Design review of the part built by this model. Coordinates are the model's own, in mm. A direction names the side the tool comes from. Give positions to 0.01 mm unless a question says otherwise; leave off trailing zeros. Loops run counter-clockwise (first coordinate to the right, second up) from the corner with the lowest first, then second, coordinate; pieces in that order, holes last.
from build123d import *

# Parameters (mm, degrees)
F0_W     = 51.3991490006
F0_H     = 50.7968105376
F0_R     = 5.0314784616
F1_DEPTH = 43.942
F2_W     = 28.5104624927
F2_H     = 18.070012331
F3_DEPTH = 25.908
F4_W     = 80.7127282023
F4_H     = 44.773478061
F5_DEPTH = 84.836


with BuildPart() as f1:
    # F0 (on Right) → F1 (new body, symmetric)
    with BuildSketch(Plane.YZ):
        with Locations((0, 25.3984052688)):
            Rectangle(F0_W, F0_H)
        with Locations((0, 25.3984052688)):
            Circle(F0_R, mode=Mode.SUBTRACT)
    extrude(amount=F1_DEPTH, both=True)

    # F2 (on Front) → F3 (cut, symmetric)
    with BuildSketch(Plane.XZ):
        with Locations((0, 41.862193495)):
            Rectangle(F2_W, F2_H)
    extrude(amount=F3_DEPTH, both=True, mode=Mode.SUBTRACT)

    # F4 (on Top) → F5 (cut)
    with BuildSketch(Plane.XY):
        Rectangle(F4_W, F4_H)
    extrude(amount=F5_DEPTH, mode=Mode.SUBTRACT)


solid = f1.part
Q1. Insertion check: pin 1 (1.7 mm diameter, centred on x = 4, y = 24.5, fed in from +Z). The pin has a flat end and moves straight along its axis. Give the tip position at first contact, or say it passes through.
Results:
pin 1: stops at z = 32.83
Q2. Take a section at D-D (y = 0). Give the boundary of the cut face in (x, z).
Results:
outline: (-43.94, 0) - (-40.36, 0) - (-40.36, 20.37) - (-43.94, 20.37) - close; (-43.94, 30.43) - (-40.36, 30.43) - (-40.36, 50.8) - (-43.94, 50.8) - close; (40.36, 0) - (43.94, 0) - (43.94, 20.37) - (40.36, 20.37) - close; (40.36, 30.43) - (43.94, 30.43) - (43.94, 50.8) - (40.36, 50.8) - close
Q3. Wall thickness on line 1 (X direction, y = -8, z = 11.5); line 2 (Y direction, x = -22.5, z = 28); line 3 (Z direction, x = -41.75, y = 0): over which ranges is each line inside the solid? List them lowest first.
Results:
line 1: x = -43.94 to -40.36, 40.36 to 43.94
line 2: y = -25.7 to -22.39, 22.39 to 25.7
line 3: z = 0 to 20.37, 30.43 to 50.8
Q4. Take a section at B-B (z = 48). Give the boundary of the cut face in (x, y).
Results:
outline: (-43.94, -25.7) - (-14.26, -25.7) - (-14.26, -22.39) - (-40.36, -22.39) - (-40.36, 22.39) - (-14.26, 22.39) - (-14.26, 25.7) - (-43.94, 25.7) - close; (14.26, -25.7) - (43.94, -25.7) - (43.94, 25.7) - (14.26, 25.7) - (14.26, 22.39) - (40.36, 22.39) - (40.36, -22.39) - (14.26, -22.39) - close
Q5. Take a section at C-C (x = 38.5). Give the boundary of the cut face in (y, z).
Results:
outline: (-25.7, 0) - (-22.39, 0) - (-22.39, 50.8) - (-25.7, 50.8) - close; (22.39, 0) - (25.7, 0) - (25.7, 50.8) - (22.39, 50.8) - close
Q6. Take a section at A-A (y = 20). Give the boundary of the cut face in (x, z), plus the area to 3 significant figures.
Results:
outline: (-43.94, 0) - (-40.36, 0) - (-40.36, 50.8) - (-43.94, 50.8) - close; (40.36, 0) - (43.94, 0) - (43.94, 50.8) - (40.36, 50.8) - close
area: 364 mm2
Q7. Draft analysis for pull direction Y (two halves, no side actions). For faces 1 (the face through (-40.356, -5.3, 25)), 2 (the face through (14.255, -24, 42)), 3 (the face through (1, -25.7, 25)), state which applies: pulls with the +Y half, pulls with the -Y half, needs draft (parallel to the pull), parting line crosses it, or undercut.
Results:
face 1: undercut
face 2: needs draft
face 3: pulls with the -Y half
Q8. Tool access review of faces 4 (the face through (1, 25.7, 25)), 5 (the face through (-1, 22.387, 25)), 6 (the face through (-14.255, 24, 42)): name each direction out of +Z, -Z, +X, -X, +Y, -Y from which nothing blocks a thin tool from reaching the whole face with its end or side.
Results:
face 4: +Z, -Z, +X, -X, +Y
face 5: +Z, -Z
face 6: +Z, +Y, -Y
